Could you check a few things on this model? Use its own coordinates, in mm. Face numbers are marked on the shaded views. A direction names the side the tool comes from. Coordinates: 2 decimals unless noted, no trailing zeros. Order: outer loops, then holes, each group sorted by start corner. A loop starts at its lowest first (then second) coordinate and runs counter-clockwise, first axis right, second up. Notation, with made-up numbers: M 82,79.25 L 141,79.25 A17 ccw 141,98.25 Z; hole C 3.25,-8.75 d2. An arc over 180 degrees is marked long. Put each result on its own line as item: value. Start each with the question number.
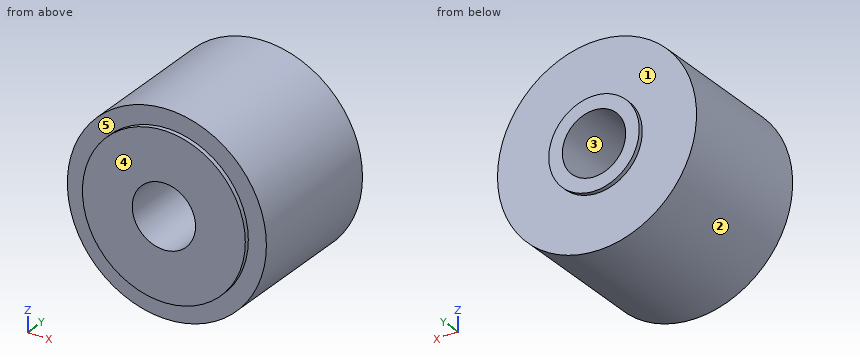
```python
from build123d import *

# Parameters (mm, degrees)
SKETCH1_R           = 11
BOSS_EXTRUDE1_DEPTH = 16
SKETCH2_R           = 5
BOSS_EXTRUDE2_DEPTH = 0.5
SKETCH3_R           = 9
BOSS_EXTRUDE3_DEPTH = 0.5
SKETCH4_R           = 3.5
CUT_EXTRUDE1_DEPTH  = 18


with BuildPart() as part:
    # Sketch1 → Boss-Extrude1 (new body)
    with BuildSketch(Plane(origin=(0, 0, 0), x_dir=(1, 0, 0), z_dir=(0, 1, 0))):
        Circle(SKETCH1_R)
    extrude(amount=BOSS_EXTRUDE1_DEPTH)

    # Sketch2 → Boss-Extrude2 (add)
    with BuildSketch(Plane(origin=(0, 16, 0), x_dir=(1, 0, 0), z_dir=(0, 1, 0))):
        Circle(SKETCH2_R)
    extrude(amount=BOSS_EXTRUDE2_DEPTH)

    # Sketch3 → Boss-Extrude3 (add)
    with BuildSketch(Plane.XZ):
        Circle(SKETCH3_R)
    extrude(amount=BOSS_EXTRUDE3_DEPTH)

    # Sketch4 → Cut-Extrude1 (cut, through all)
    with BuildSketch(Plane(origin=(0, 16.5, 0), x_dir=(1, 0, 0), z_dir=(0, 1, 0))):
        Circle(SKETCH4_R)
    extrude(amount=-CUT_EXTRUDE1_DEPTH, mode=Mode.SUBTRACT)


solid = part.part
```
Item 1: If we section it at A-A on x = 0: Write out the boundary of the cut face in (y, z).
Item 2: If we mould it in two halves opening along Z, with no side actions, what happens to the marked faces 1, 2 and 3? For each: released by +Z, released by -Z, zero draft, split by the parting line, or undercut.
Item 3: If we section it at B-B on z = 0: Write out the boundary of the cut face in (x, y).
Item 4: For pin 1 Ø10 at (x, z) = (5, 4) entering from +Y; pin 2 Ø5 at (y, z) = (7, -3) entering from +X; pin 3 Ø3 at (y, z) = (14.5, -7.5) entering from +X; pin 4 Ø6.5 at (x, z) = (0, 0) entering from -Y, each with a flat end and sliding along its axis, tell me the tip position at first contact or that it passes through.
Item 5: I need wall thicknesses on probe 1 along Z at (x, y) = (0, 9.25); probe 2 along Y at (x, z) = (-6.75, -3). Which ranges of each line are inside material? Lowest first, please.
Item 6: If we section it at D-D on z = 5.75: Write out the boundary of the cut face in (x, y), then the cut area to 3 significant figures.
Item 7: If we section it at C-C on y = 13.75: Write out the boundary of the cut face in (x, z), then the cut area to 3 significant figures.
Item 8: For the marked faces 4 and 5, which set-ups out of +Z, -Z, +X, -X, +Y, -Y let a thin tool reach every point of the face, with its end or its side?
Geometry check:
1. outline: M -0.5,-9 L 0,-9 L 0,-11 L 16,-11 L 16,-5 L 16.5,-5 L 16.5,-3.5 L -0.5,-3.5 Z; M -0.5,3.5 L 16.5,3.5 L 16.5,5 L 16,5 L 16,11 L 0,11 L 0,9 L -0.5,9 Z
2. face 1: zero draft
2. face 2: split by the parting line
2. face 3: undercut
3. outline: M -11,0 L -9,0 L -9,-0.5 L -3.5,-0.5 L -3.5,16.5 L -5,16.5 L -5,16 L -11,16 Z; M 3.5,-0.5 L 9,-0.5 L 9,0 L 11,0 L 11,16 L 5,16 L 5,16.5 L 3.5,16.5 Z
4. pin 1: stops at y = 16.5
4. pin 2: stops at x = 10.99
4. pin 3: stops at x = 9.22
4. pin 4: passes through
5. probe 1: z = -11 to -3.5, 3.5 to 11
5. probe 2: y = -0.5 to 16
6. outline: M -9.38,0 L -6.92,0 L -6.92,-0.5 L 6.92,-0.5 L 6.92,0 L 9.38,0 L 9.38,16 L -9.38,16 Z
6. area: 307 mm²
7. outline: C 0,0 d22; hole C 0,0 d7
7. area: 342 mm²
8. face 4: +Z, -Z, +X, -X, -Y
8. face 5: -Y
